The listing builds one solid part. Answer for the finished solid, in the listing's coordinates (mm). A direction names the side the tool comes from. Round coordinates to 2 decimals unless told otherwise and drop trailing zeros. Write each loop counter-clockwise with the first axis right and the second up, starting at its lowest first coordinate (ties: lowest second). Pieces come first, ordered by that corner, then holes.
Item 1: Find section C-C on y = 5.25. Give the number of separate pieces and of enclosed holes in the cut face, then the cut area to 3 significant figures.
Item 2: A tool of negligible diameter and unlimited length cuts with its end or side. For faces 4 (the face through (37.24, 3.13, -193.56)), 5 (the face through (6.76, 3.22, -468.04)), from which of +Z, -Z, +X, -X, +Y, -Y can it reach the whole face along a straight path? Write none if from no direction.
Item 3: Find section A-A on z = -222. Give the vertices of the cut face in (x, y).
Item 4: Find section B-B on x = 202. Give the vertices of the cut face in (y, z).
Item 5: For a pull along Z with two mould halves and no side action, classify faces 1 (the face through (125, 0, -250)), 2 (the face through (195.753, 3.219, -493.414)), 3 (the face through (61.275, 3.131, -34.086)) as +Z half, -Z half, draft (parallel to the pull), parting line (faces both ways), or undercut.
Item 6: Find the intervals of material crossed by probe 1 along X at (y, z) = (1.5, -40); probe 2 along Z at (x, y) = (30, 2.25); probe 3 along X at (y, z) = (1.75, -336), in increasing order.
Item 7: Each of these flat-tipped pins is pushed along its axis until it touches: pin 1 (2 mm diameter, centred on y = 5.5, z = -167, fed in from +X); pin 2 (1 mm diameter, centred on y = 4, z = -417.5, fed in from -X); pin 3 (1.9 mm diameter, centred on x = -4.5, y = 1.5, fed in from -Z). Where does it stop, or does it pass through?
```python
from build123d import *

# Parameters (mm, degrees)
SKETCH2_W           = 254
SKETCH2_H           = 508
SKETCH2_R           = 11
SKETCH2_R_2         = 1.5
SKETCH2_R_3         = 5
SKETCH2_R_4         = 2
SKETCH2_W_2         = 12.25
SKETCH2_H_2         = 22.45
BOSS_EXTRUDE1_DEPTH = 6.35
CUT_EXTRUDE1_REACH  = 569.997
CUT_EXTRUDE2_REACH  = 569.997
SKETCH7_W           = 6.35
SKETCH7_H           = 50.8
BOSS_EXTRUDE2_DEPTH = 6.35
LPATTERN1_COUNT     = 4
LPATTERN1_PITCH     = 101.6
CUT_EXTRUDE3_REACH  = 572.865
SKETCH8_W           = 6.35
SKETCH8_H           = 50.8
LPATTERN2_COUNT     = 3
LPATTERN2_PITCH     = 101.6


with BuildPart() as part:
    # Sketch2 → Boss-Extrude1 (new body)
    with BuildSketch(Plane(origin=(0, 0, 0), x_dir=(1, 0, 0), z_dir=(0, 1, 0))):
        with Locations((127, 254)):
            Rectangle(SKETCH2_W, SKETCH2_H)
        with Locations(Location((52, 40, 0), (0, 0, 270))):
            Circle(SKETCH2_R, mode=Mode.SUBTRACT)
        with Locations(Location((202, 40, 0), (0, 0, 90))):
            Circle(SKETCH2_R, mode=Mode.SUBTRACT)
        with Locations(Location((38.246918035, 45.332917816, 0), (0, 0, 270))):
            Circle(SKETCH2_R_2, mode=Mode.SUBTRACT)
        with Locations(Location((34.015423002, 186.409908658, 0), (0, 0, 270))):
            Circle(SKETCH2_R_3, mode=Mode.SUBTRACT)
        with Locations(Location((57.09109314, 362.75, 0), (0, 0, 270))):
            Circle(SKETCH2_R_2, mode=Mode.SUBTRACT)
        with Locations(Location((184.628948138, 428.795408939, 0), (0, 0, 270))):
            Circle(SKETCH2_R_4, mode=Mode.SUBTRACT)
        with Locations(Location((146.628948138, 428.795408939, 0), (0, 0, 270))):
            Circle(SKETCH2_R_4, mode=Mode.SUBTRACT)
        with Locations(Location((139.628948138, 428.795408939, 0), (0, 0, 270))):
            Circle(SKETCH2_R_4, mode=Mode.SUBTRACT)
        with Locations(Location((101.628948138, 428.795408939, 0), (0, 0, 270))):
            Circle(SKETCH2_R_4, mode=Mode.SUBTRACT)
        with BuildLine():
            Line((3.046441744, 262.929522506), (8.097429065, 262.929522506))
            add(Edge.make_bspline(
                [(8.097429065, 262.929522506), (9.552300843, 252.9110337), (11.964991372, 242.951994092), (16.119595939, 233.68781707)],
                knots=[0, 0, 0, 0, 1, 1, 1, 1], degree=3))
            Line((16.119595939, 233.68781707), (12.017665952, 230.63111289))
            add(Edge.make_bspline(
                [(3.046441744, 262.929522506), (4.60754392, 251.841244803), (7.285656471, 240.828405001), (12.017665952, 230.63111289)],
                knots=[0, 0, 0, 0, 1, 1, 1, 1], degree=3))
        make_face(mode=Mode.SUBTRACT)
        Polygon((31.329859517, 200.915527121), (35.257076266, 204.010194891), (46.889107588, 189.528125605), (42.980562709, 186.409908658), align=None, mode=Mode.SUBTRACT)
        with Locations((33.940423002, 160.784908658)):
            Rectangle(SKETCH2_W_2, SKETCH2_H_2, mode=Mode.SUBTRACT)
        with BuildLine():
            Line((138.65, 474.05), (138.65, 467.05))
            add(Edge.make_bspline(
                [(138.65, 467.05), (138.65, 464.55), (143.65, 464.55), (148.65, 464.55), (148.65, 467.05)],
                knots=[0, 0, 0, 1.570796327, 1.570796327, 3.141592654, 3.141592654, 3.141592654], degree=2, weights=[1, 0.707106781, 1, 0.707106781, 1]))
            Line((148.65, 467.05), (148.65, 474.05))
            add(Edge.make_bspline(
                [(148.65, 474.05), (148.65, 476.55), (143.65, 476.55), (138.65, 476.55), (138.65, 474.05)],
                knots=[3.141592654, 3.141592654, 3.141592654, 4.71238898, 4.71238898, 6.283185307, 6.283185307, 6.283185307], degree=2, weights=[1, 0.707106781, 1, 0.707106781, 1]))
        make_face(mode=Mode.SUBTRACT)
        with BuildLine():
            Line((63.65, 447.05), (63.65, 454.05))
            add(Edge.make_bspline(
                [(63.65, 454.05), (63.65, 456.55), (58.65, 456.55), (53.65, 456.55), (53.65, 454.05)],
                knots=[0, 0, 0, 1.570796327, 1.570796327, 3.141592654, 3.141592654, 3.141592654], degree=2, weights=[1, 0.707106781, 1, 0.707106781, 1]))
            Line((53.65, 454.05), (53.65, 447.05))
            add(Edge.make_bspline(
                [(53.65, 447.05), (53.65, 444.55), (58.65, 444.55), (63.65, 444.55), (63.65, 447.05)],
                knots=[3.141592654, 3.141592654, 3.141592654, 4.71238898, 4.71238898, 6.283185307, 6.283185307, 6.283185307], degree=2, weights=[1, 0.707106781, 1, 0.707106781, 1]))
        make_face(mode=Mode.SUBTRACT)
        with BuildLine():
            ThreePointArc((33.415423002, 175.759908658), (34.015423002, 173.959908658), (34.615423002, 175.759908658))
            ThreePointArc((34.615423002, 175.759908658), (34.015423002, 175.959908658), (33.415423002, 175.759908658))
        make_face(mode=Mode.SUBTRACT)
        with BuildLine():
            ThreePointArc((34.615423002, 145.659908658), (34.015423002, 147.459908658), (33.415423002, 145.659908658))
            ThreePointArc((33.415423002, 145.659908658), (34.015423002, 145.459908658), (34.615423002, 145.659908658))
        make_face(mode=Mode.SUBTRACT)
    extrude(amount=BOSS_EXTRUDE1_DEPTH)

    # Sketch3 → Cut-Extrude1 (cut, up to next)
    with BuildSketch(Plane(origin=(0, 6.35, 0), x_dir=(1, 0, 0), z_dir=(0, 1, 0)), mode=Mode.PRIVATE) as cut_extrude1_sk1:
        with BuildLine():
            Line((254, 508), (127, 508))
            ThreePointArc((127, 508), (196.670138835, 493.003472168), (254, 450.670138835))
            Line((254, 450.670138835), (254, 508))
        make_face()
    cut_extrude1_tool1 = extrude(cut_extrude1_sk1.sketch, amount=-CUT_EXTRUDE1_REACH, mode=Mode.PRIVATE) & part.part
    add(cut_extrude1_tool1.solids().sort_by_distance((223.425214, 6.35, -491.44845))[0], mode=Mode.SUBTRACT)

    # Sketch5 → Cut-Extrude2 (cut, up to next)
    with BuildSketch(Plane(origin=(0, 6.35, 0), x_dir=(1, 0, 0), z_dir=(0, 1, 0)), mode=Mode.PRIVATE) as cut_extrude2_sk1:
        with BuildLine():
            Line((3, 450.670138835), (0, 445.807083784))
            Line((0, 445.807083784), (0, 508))
            Line((0, 508), (0, 526.766169575))
            Line((0, 526.766169575), (127, 526.766169575))
            Line((127, 526.766169575), (127, 508))
            add(Edge.make_bspline(
                [(16.993362097, 481.969152132), (44.771100023, 511.766098677), (91.209279055, 505.856564635), (127, 508)],
                knots=[0, 0, 0, 0, 1, 1, 1, 1], degree=3))
            ThreePointArc((16.993362097, 481.969152132), (6.657603153, 467.812501684), (3, 450.670138835))
        make_face()
    cut_extrude2_tool1 = extrude(cut_extrude2_sk1.sketch, amount=-CUT_EXTRUDE2_REACH, mode=Mode.PRIVATE) & part.part
    add(cut_extrude2_tool1.solids().sort_by_distance((49.030169, 6.35, -509.000401))[0], mode=Mode.SUBTRACT)

    # Sketch7 → Boss-Extrude2 (add)
    with BuildSketch(Plane.XZ):
        with Locations((257.175, -25.4)):
            Rectangle(SKETCH7_W, SKETCH7_H)
        with Locations((-3.175, -25.4)):
            Rectangle(SKETCH7_W, SKETCH7_H)
    boss_extrude2 = extrude(amount=-BOSS_EXTRUDE2_DEPTH)

    # LPattern1: Boss-Extrude2 ×4
    with Locations(*[(0, 0, -i * LPATTERN1_PITCH) for i in range(1, LPATTERN1_COUNT)]):
        add(boss_extrude2)

    # Sketch8 → Cut-Extrude3 (cut, up to next)
    with BuildSketch(Plane(origin=(0, 6.35, 0), x_dir=(1, 0, 0), z_dir=(0, 1, 0)), mode=Mode.PRIVATE) as cut_extrude3_sk1:
        with Locations((230.825, 127)):
            Rectangle(SKETCH8_W, SKETCH8_H)
    cut_extrude3_tool1 = extrude(cut_extrude3_sk1.sketch, amount=-CUT_EXTRUDE3_REACH, mode=Mode.PRIVATE) & part.part
    cut_extrude3 = cut_extrude3_tool1.solids().sort_by_distance((230.825, 6.35, -127))[0]
    add(cut_extrude3, mode=Mode.SUBTRACT)

    # LPattern2: Cut-Extrude3 ×3
    with Locations(*[(0, 0, -i * LPATTERN2_PITCH) for i in range(1, LPATTERN2_COUNT)]):
        add(cut_extrude3, mode=Mode.SUBTRACT)


solid = part.part
```
Check values:
1. separate pieces: 1
1. enclosed holes: 19
1. area: 125,000 mm2
2. face 4: +Y, -Y
2. face 5: -Z, -X, +Y, -Y
3. outline: (-6.35, 0) - (227.65, 0) - (227.65, 6.35) - (-6.35, 6.35) - close; (234, 0) - (260.35, 0) - (260.35, 6.35) - (234, 6.35) - close
4. outline: (0, -490.48) - (6.35, -490.48) - (6.35, -51) - (0, -51) - close; (0, -29) - (6.35, -29) - (6.35, 0) - (0, 0) - close
5. face 1: draft
5. face 2: -Z half
5. face 3: undercut
6. probe 1: x = -6.35 to 41, 63 to 191, 213 to 260.35
6. probe 2: z = -492.71 to -189.39, -183.43 to -172.01, -149.56 to 0
6. probe 3: x = -6.35 to 227.65, 234 to 260.35
7. pin 1: stops at x = 254
7. pin 2: stops at x = 0
7. pin 3: stops at z = -355.6
